from build123d import *

# Parameters (mm, degrees)
SKETCH1_R           = 15
SKETCH1_W           = 523.453034516
SKETCH1_H           = 6
BOSS_EXTRUDE1_DEPTH = 6


with BuildPart() as part:
    # Sketch1 → Boss-Extrude1 (new body)
    with BuildSketch(Plane.YZ):
        with BuildLine():
            Line((-165.811435327, 45.958456005), (-165.811435327, 10.958456005))
            Line((-165.811435327, 10.958456005), (-159.811435327, 10.958456005))
            Line((-159.811435327, 10.958456005), (-159.811435327, -29.041543995))
            Line((-159.811435327, -29.041543995), (-165.811435327, -29.041543995))
            Line((-165.811435327, -29.041543995), (-165.811435327, -54.041543995))
            Line((-165.811435327, -54.041543995), (-159.811435327, -54.041543995))
            Line((-159.811435327, -54.041543995), (-159.811435327, -94.041543995))
            Line((-159.811435327, -94.041543995), (-165.811435327, -94.041543995))
            Line((-165.811435327, -94.041543995), (-165.811435327, -113.496690816))
            Line((-165.811435327, -113.496690816), (-125.811435327, -113.496690816))
            Line((-125.811435327, -113.496690816), (-125.811435327, -108.496690816))
            ThreePointArc((-125.811435327, -108.496690816), (-124.346969233, -104.96115691), (-120.811435327, -103.496690816))
            Line((-120.811435327, -103.496690816), (388.788564673, -103.496690816))
            ThreePointArc((388.788564673, -103.496690816), (392.324098579, -104.96115691), (393.788564673, -108.496690816))
            Line((393.788564673, -108.496690816), (393.788564673, -113.496690816))
            Line((393.788564673, -113.496690816), (443.788564673, -113.496690816))
            Line((443.788564673, -113.496690816), (443.788564673, -23.496690816))
            Line((443.788564673, -23.496690816), (-165.811435327, 45.958456005))
        make_face()
        with Locations(Location((308.788564673, -63.496690816, 0), (0, 0, 270))):
            Circle(SKETCH1_R, mode=Mode.SUBTRACT)
        Polygon((-117.76145538, 20.354457657), (-118.440674663, 14.393026523), (416.988579422, -46.611431244), (417.667798704, -40.65000011), align=None, mode=Mode.SUBTRACT)
        with Locations((149.276829124, -90.496690816)):
            Rectangle(SKETCH1_W, SKETCH1_H, mode=Mode.SUBTRACT)
    extrude(amount=BOSS_EXTRUDE1_DEPTH)


solid = part.part
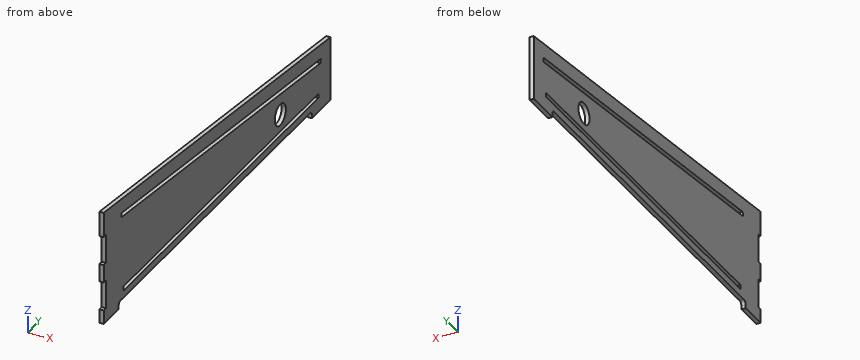
The model under review builds one solid part; all positions refer to its coordinate system, in mm. Give positions to 0.01 mm unless a question says otherwise; leave off trailing zeros. Loops run counter-clockwise (first coordinate to the right, second up) from the corner with the lowest first, then second, coordinate; pieces in that order, holes last. Notation, with made-up numbers: (39, 65) -> (74, 65) arc R14 ccw to (74, 89) -> close; hole circle Ø8 at (25.25, 82). An arc over 180 degrees is marked (long way). Put each result on its own line as item: value. Start each with the question number.
1. We need section A-A on z = -2.5. State the section outline as (x, y) points.
2. We need section B-B on y = 35.5. State the section outline as (x, z) points.
3. We need section C-C on x = 3.05. State the section outline as (y, z) points, then the cut area to 3 significant figures.
4. We need section D-D on y = 221. State the section outline as (x, z) points.
5. Wall thickness on probe 1 along Z at (x, y) = (3.25, -94); probe 2 along Z at (x, y) = (2.3, 78); probe 3 along Y at (x, z) = (2.7, -63.5): over which ranges is each line inside the solid? List them lowest first.
6. Clearance check with flat-ended pins moving along their axes: P1, Ø1.5, axis at x = 5, z = -57.5, coming from the -Y side; P2, Ø3, axis at x = 3, y = -161.5, coming from the +Z side; P3, Ø1.8, axis at x = 4, y = 108.5, coming from the -Z side. State where each tip first meets the part, or that it passes through.
Determined:
1. outline: (0, -159.81) -> (6, -159.81) -> (6, 29.83) -> (0, 29.83) -> close; (0, 82.83) -> (6, 82.83) -> (6, 259.5) -> (0, 259.5) -> close
2. outline: (0, -103.5) -> (6, -103.5) -> (6, -93.5) -> (0, -93.5) -> close; (0, -87.5) -> (6, -87.5) -> (6, -3.15) -> (0, -3.15) -> close; (0, 2.89) -> (6, 2.89) -> (6, 23.02) -> (0, 23.02) -> close
3. outline: (-165.81, -113.5) -> (-125.81, -113.5) -> (-125.81, -108.5) arc R5 cw to (-120.81, -103.5) -> (388.79, -103.5) arc R5 cw to (393.79, -108.5) -> (393.79, -113.5) -> (443.79, -113.5) -> (443.79, -23.5) -> (-165.81, 45.96) -> (-165.81, 10.96) -> (-159.81, 10.96) -> (-159.81, -29.04) -> (-165.81, -29.04) -> (-165.81, -54.04) -> (-159.81, -54.04) -> (-159.81, -94.04) -> (-165.81, -94.04) -> close; hole (-118.44, 14.39) -> (416.99, -46.61) -> (417.67, -40.65) -> (-117.76, 20.35) -> close; hole (-112.45, -93.5) -> (411, -93.5) -> (411, -87.5) -> (-112.45, -87.5) -> close; hole circle Ø30 at (308.79, -63.5)
3. area: 63,300 mm^2
4. outline: (0, -103.5) -> (6, -103.5) -> (6, -93.5) -> (0, -93.5) -> close; (0, -87.5) -> (6, -87.5) -> (6, -24.28) -> (0, -24.28) -> close; (0, -18.24) -> (6, -18.24) -> (6, 1.89) -> (0, 1.89) -> close
5. probe 1: -103.5 to -93.5, -87.5 to 11.61, 17.65 to 37.78
5. probe 2: -103.5 to -93.5, -87.5 to -7.99, -1.95 to 18.18
5. probe 3: -159.81 to 293.79, 323.79 to 443.79
6. P1: y = -159.81
6. P2: z = 45.64
6. P3: z = -103.5
